Input: part model. Units: mm. Frame: model coordinates. A direction names the side the tool comes from. Coordinates: 2 decimals unless noted, no trailing zeros. Loops run counter-clockwise (first coordinate to the right, second up) from the corner with the lowest first, then second, coordinate; pieces in that order, holes last. Notation, with made-up numbers: (1, 79.5) -> (18, 79.5) arc R18 cw to (18, 88.5) -> close; hole circle Ø10 at (45.5, 38.25). An arc over 180 degrees is marked (long way). Answer as a JSON object with one key per item and string values.
from build123d import *

# Parameters (mm, degrees)
F1_DEPTH = 17.2
F2_R     = 1.5
F3_DEPTH = 1.2
F5_DEPTH = 1.2


# Not quite as in the source:
# - a fillet or chamfer that OpenCascade refuses, or shapes differently, is made with other operations: its cross-section is extruded or revolved along the edge and cut away or added


with BuildPart() as f1:
    # F0 (on Front) → F1 (new body)
    with BuildSketch(Plane.XZ):
        with BuildLine():
            Line((-20.1, 5.7260450742), (-22.1961550602, 17.6139311585))
            ThreePointArc((-22.1961550602, 17.6139311585), (-22.4238939618, 19.3437798569), (-22.5, 21.0868947118))
            Line((-22.5, 21.0868947118), (-22.5, 27))
            Line((-22.5, 27), (-24.1, 27))
            Line((-24.1, 27), (-24.1, 21.0868947118))
            ThreePointArc((-24.1, 21.0868947118), (-24.0178054788, 19.2043306685), (-23.7718474651, 17.3360940742))
            Line((-23.7718474651, 17.3360940742), (-21.6756924048, 5.44820799))
            ThreePointArc((-21.6756924048, 5.44820799), (-19.7066672631, 1.205023255), (-15.889887542, -1.4993933668))
            ThreePointArc((-15.889887542, -1.4993933668), (0, -4.3622248316), (15.889887542, -1.4993933668))
            ThreePointArc((15.889887542, -1.4993933668), (19.7066672631, 1.205023255), (21.6756924048, 5.44820799))
            Line((21.6756924048, 5.44820799), (23.7718474651, 17.3360940742))
            ThreePointArc((23.7718474651, 17.3360940742), (24.0178054788, 19.2043306685), (24.1, 21.0868947118))
            Line((24.1, 21.0868947118), (24.1, 27))
            Line((24.1, 27), (22.5, 27))
            Line((22.5, 27), (22.5, 21.0868947118))
            ThreePointArc((22.5, 21.0868947118), (22.4238939618, 19.3437798569), (22.1961550602, 17.6139311585))
            Line((22.1961550602, 17.6139311585), (20.1, 5.7260450742))
            ThreePointArc((20.1, 5.7260450742), (18.477177081, 2.2289147982), (15.3314795087, 0))
            ThreePointArc((15.3314795087, 0), (0, -2.7622248316), (-15.3314795087, 0))
            ThreePointArc((-15.3314795087, 0), (-18.477177081, 2.2289147982), (-20.1, 5.7260450742))
        make_face()
    extrude(amount=F1_DEPTH)

    # F2 (on face) → F3 (join)
    with BuildSketch(Plane.XZ.offset(17.2)):
        with BuildLine():
            Line((24.1, 27), (-24.1, 27))
            Line((-24.1, 27), (-24.1, 21.0868947118))
            ThreePointArc((-24.1, 21.0868947118), (-24.0178054788, 19.2043306685), (-23.7718474651, 17.3360940742))
            Line((-23.7718474651, 17.3360940742), (-21.6756924048, 5.44820799))
            ThreePointArc((-21.6756924048, 5.44820799), (-19.7066672631, 1.205023255), (-15.889887542, -1.4993933668))
            ThreePointArc((-15.889887542, -1.4993933668), (0, -4.3622248316), (15.889887542, -1.4993933668))
            ThreePointArc((15.889887542, -1.4993933668), (19.7066672631, 1.205023255), (21.6756924048, 5.44820799))
            Line((21.6756924048, 5.44820799), (23.7718474651, 17.3360940742))
            ThreePointArc((23.7718474651, 17.3360940742), (24.0178054788, 19.2043306685), (24.1, 21.0868947118))
            Line((24.1, 21.0868947118), (24.1, 27))
        make_face()
        with Locations((0, 18)):
            Circle(F2_R, mode=Mode.SUBTRACT)
    extrude(amount=F3_DEPTH)

    # F4 (on face) → F5 (join)
    with BuildSketch(Plane(origin=(0, 0, 0), x_dir=(-1, 0, 0), z_dir=(0, 1, 0))):
        with BuildLine():
            Line((-24.1, 27), (-24.1, 21.0868947118))
            ThreePointArc((-24.1, 21.0868947118), (-24.0178054788, 19.2043306685), (-23.7718474651, 17.3360940742))
            Line((-23.7718474651, 17.3360940742), (-21.6756924048, 5.44820799))
            ThreePointArc((-21.6756924048, 5.44820799), (-19.7066672631, 1.205023255), (-15.889887542, -1.4993933668))
            ThreePointArc((-15.889887542, -1.4993933668), (0, -4.3622248316), (15.889887542, -1.4993933668))
            ThreePointArc((15.889887542, -1.4993933668), (19.7066672631, 1.205023255), (21.6756924048, 5.44820799))
            Line((21.6756924048, 5.44820799), (23.7718474651, 17.3360940742))
            ThreePointArc((23.7718474651, 17.3360940742), (24.0178054788, 19.2043306685), (24.1, 21.0868947118))
            Line((24.1, 21.0868947118), (24.1, 27))
            Line((24.1, 27), (17.5, 27))
            Line((17.5, 27), (17.5, 21.0868947118))
            ThreePointArc((17.5, 21.0868947118), (17.4429204714, 19.7795585706), (17.2721162952, 18.4821720468))
            Line((17.2721162952, 18.4821720468), (15.1759612349, 6.5942859626))
            ThreePointArc((15.1759612349, 6.5942859626), (14.6350202619, 5.4285758705), (13.5864544045, 4.6856042711))
            ThreePointArc((13.5864544045, 4.6856042711), (0, 2.2377751684), (-13.5864544045, 4.6856042711))
            ThreePointArc((-13.5864544045, 4.6856042711), (-14.6350202619, 5.4285758705), (-15.1759612349, 6.5942859626))
            Line((-15.1759612349, 6.5942859626), (-17.2721162952, 18.4821720468))
            ThreePointArc((-17.2721162952, 18.4821720468), (-17.4429204714, 19.7795585706), (-17.5, 21.0868947118))
            Line((-17.5, 21.0868947118), (-17.5, 27))
            Line((-17.5, 27), (-24.1, 27))
        make_face()
    extrude(amount=F5_DEPTH)

    # F6: chamfer of 2 on 1 edges, made by hand

    # F6_s1 → F6_t2 (revolve, cut)
    with BuildSketch(Plane.XY.offset(18)):
        Polygon((3.5, -17.2), (1.5, -19.2), (1.5, -17.2), align=None)
    revolve(axis=Axis((0, -17.2, 18), (0, -1, 0)), mode=Mode.SUBTRACT)


solid = f1.part
1. Mould query, pull axis Y, two halves, no side actions, for faces 1 (the face through (-22.42, -8.48, 19.32)), 2 (the face through (21.163, -8.48, 11.753)), 3 (the face through (17.5, 1, 24)). Classes: pulls with the +Y half, pulls with the -Y half, needs draft (parallel to the pull), parting line crosses it, or undercut.
Reply:
{"face 1": "undercut", "face 2": "undercut", "face 3": "needs draft"}
2. Pin query (flat end, axial travel): P1, Ø10, axis at x = -7.5, y = -11, coming from the +Z side; P2, Ø8, axis at x = 2.5, y = -12.5, coming from the +Z side; P3, Ø3, axis at x = 1, y = -12, coming from the +Z side. Return the tip coordinate at first contact, or that it passes through.
Reply:
{"P1": "stops at z = -0.95", "P2": "stops at z = -2.28", "P3": "stops at z = -2.69"}
3. Section query C-C (z = 24.5). Return loops of the section in (x, y).
Reply:
{"outline": "(-24.1, -18.4) -> (24.1, -18.4) -> (24.1, 1.2) -> (17.5, 1.2) -> (17.5, 0) -> (22.5, 0) -> (22.5, -17.2) -> (-22.5, -17.2) -> (-22.5, 0) -> (-17.5, 0) -> (-17.5, 1.2) -> (-24.1, 1.2) -> close"}
4. Access query for faces 4 (the face through (24.1, -9, 24)), 5 (the face through (-18.442, -8.48, 2.187)), 6 (the face through (-0.19, 0.59, 2.24)). Directions: +Z, -Z, +X, -X, +Y, -Y. A direction counts if a zero-diameter tool reaches every point of the face in a straight line with its end or side. Return the directions, or none.
Reply:
{"face 4": "+Z, -Z, +X, +Y, -Y", "face 5": "+Z", "face 6": "+Z, +Y"}
5. Line query: line 1 along X through (y, z) = (-3.5, 22.5); line 2 along Y through (x, z) = (21, 20); line 3 along Y through (x, z) = (9, 12). Output: solid intervals per line, ascending.
Reply:
{"line 1": "x = -24.1 to -22.5, 22.5 to 24.1", "line 2": "y = -18.4 to -17.2, 0 to 1.2", "line 3": "y = -18.4 to -17.2"}
6. Section query A-A (x = 0). Return loops of the section in (y, z), plus the area to 3 significant figures.
Reply:
{"outline": "(-18.4, -4.36) -> (1.2, -4.36) -> (1.2, 2.24) -> (0, 2.24) -> (0, -2.76) -> (-17.2, -2.76) -> (-17.2, 14.5) -> (-18.4, 15.7) -> close; (-18.4, 20.3) -> (-17.2, 21.5) -> (-17.2, 27) -> (-18.4, 27) -> close", "area": "66.1 mm2"}
7. Section query B-B (y = -9.5). Return loops of the section in (x, z).
Reply:
{"outline": "(-24.1, 21.09) arc R21.6 ccw to (-23.77, 17.34) -> (-21.68, 5.45) arc R9.1 ccw to (-15.89, -1.5) arc R45.53 ccw to (15.89, -1.5) arc R9.1 ccw to (21.68, 5.45) -> (23.77, 17.34) arc R21.6 ccw to (24.1, 21.09) -> (24.1, 27) -> (22.5, 27) -> (22.5, 21.09) arc R20 cw to (22.2, 17.61) -> (20.1, 5.73) arc R7.5 cw to (15.33, 0) arc R43.93 cw to (-15.33, 0) arc R7.5 cw to (-20.1, 5.73) -> (-22.2, 17.61) arc R20 cw to (-22.5, 21.09) -> (-22.5, 27) -> (-24.1, 27) -> close"}
8. Section query D-D (x = 10). Return loops of the section in (y, z).
Reply:
{"outline": "(-18.4, -3.25) -> (1.2, -3.25) -> (1.2, 3.54) -> (0, 3.54) -> (0, -1.61) -> (-17.2, -1.61) -> (-17.2, 27) -> (-18.4, 27) -> close"}
